For this review, take the finished solid that the model builds, in its own axes (mm). Face numbers are marked on the shaded views. Give positions to 0.01 mm unless a question says otherwise; leave off trailing zeros. Loops run counter-clockwise (first coordinate to the right, second up) from the corner with the lowest first, then second, coordinate; pieces in that order, holes last.
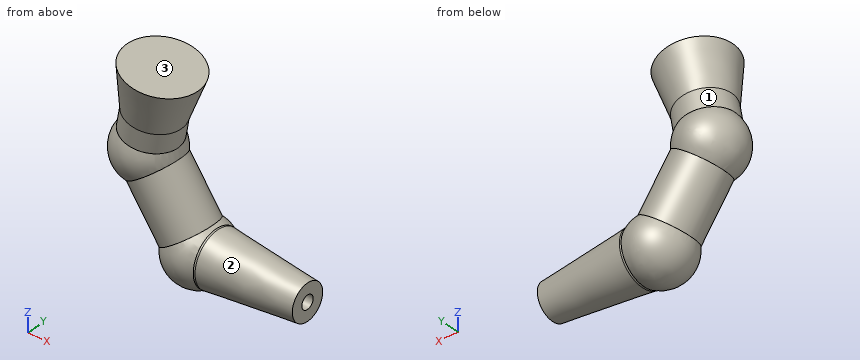
```python
from build123d import *

# Parameters (mm, degrees)
ESQUISSE1_R        = 3
ESQUISSE1_R_2      = 0.75
BOSS_EXTRU_1_DEPTH = 12
CHANFREIN1_SIZE    = 10
CHANFREIN1_SIZE2   = 1
ESQUISSE4_R        = 3
BOSS_EXTRU_2_DEPTH = 10
ESQUISSE8_R        = 3
BOSS_EXTRU_3_DEPTH = 4
ESQUISSE10_R       = 4
BOSS_EXTRU_4_DEPTH = 5
CHANFREIN2_SIZE    = 5
CHANFREIN2_SIZE_2  = 1


with BuildPart() as part:
    # Esquisse1 → Boss.-Extru.1 (new body)
    with BuildSketch(Plane(origin=(0, 0, 0), x_dir=(0, 0, -1), z_dir=(1, 0, 0))):
        Circle(ESQUISSE1_R)
        Circle(ESQUISSE1_R_2, mode=Mode.SUBTRACT)
    extrude(amount=BOSS_EXTRU_1_DEPTH)

    # Chanfrein1
    chanfrein1_edges = [part.edges().sort_by_distance(p)[0] for p in [
        (12, 0, 3),
    ]]
    chanfrein1_side = [part.faces().sort_by_distance(p)[0] for p in [
        (6, 0, 3),
    ]]
    chamfer(chanfrein1_edges, length=CHANFREIN1_SIZE, length2=CHANFREIN1_SIZE2, reference=chanfrein1_side[0])

    # Esquisse2 → Révolution1 (revolve)
    with BuildSketch(Plane.ZY):
        with BuildLine():
            Line((0, 3.5), (0, -3.5))
            ThreePointArc((0, -3.5), (-3.5, 0), (0, 3.5))
        make_face()
    revolve(axis=Axis((0, 3.5, 0), (0, -1, 0)))

    # Esquisse4 → Boss.-Extru.2 (add)
    with BuildSketch(Plane(origin=(0, 0, 0), x_dir=(0, 1, 0), z_dir=(-0.5735764363510443, 0, 0.819152044288993))):
        with Locations(Location((0, 0, 0), (0, 0, 90))):
            Circle(ESQUISSE4_R)
    extrude(amount=BOSS_EXTRU_2_DEPTH)

    # Esquisse7 → Révolution2 (revolve)
    with BuildSketch(Plane(origin=(-5.735764364, 0, 8.191520443), x_dir=(0.8191520442889931, 0, 0.5735764363510444), z_dir=(-0.5735764363510444, 0, 0.8191520442889931))):
        with BuildLine():
            Line((0, 3.5), (0, -3.5))
            ThreePointArc((0, -3.5), (-3.5, 0), (0, 3.5))
        make_face()
    revolve(axis=Axis((-5.735764364, -5.88356871, 8.191520443), (0, 1, 0)))

    # Esquisse8 → Boss.-Extru.3 (add)
    with BuildSketch(Plane(origin=(1.22787804, 0, 6.963642403), x_dir=(0, 1, 0), z_dir=(0.1736481776669342, 0, 0.9848077530122075))):
        with Locations(Location((0, 7.071067812, 0), (0, 0, 90))):
            Circle(ESQUISSE8_R)
    extrude(amount=BOSS_EXTRU_3_DEPTH)

    # Esquisse10 → Boss.-Extru.4 (add)
    with BuildSketch(Plane(origin=(1.92247075, 0, 10.902873415), x_dir=(0.9848077530122075, 0, -0.17364817766693422), z_dir=(0.17364817766693422, 0, 0.9848077530122075))):
        with Locations((-7.071067812, 0)):
            Circle(ESQUISSE10_R)
    extrude(amount=BOSS_EXTRU_4_DEPTH)

    # Chanfrein2
    # the kernel refuses this chamfer: 5, 1 mm, written as the material it takes off along each edge
    with BuildSketch(Plane(origin=(-5.041171653, 0, 12.130751455), x_dir=(0.9848077530122075, 0, -0.17364817766693408), z_dir=(0, -1, 0))) as chanfrein2_piece_1:
        Polygon((4, CHANFREIN2_SIZE), (4 - CHANFREIN2_SIZE_2, 0), (4, 0), align=None)
    revolve(axis=Axis((-5.041171653, 0, 12.130751455), (0.17364817766693422, 0, 0.9848077530122075)), mode=Mode.SUBTRACT)


solid = part.part
```
Item 1: The part is to be moulded in two halves that separate along Z. For the marked faces 1, 2 and 3, say which applies: released by +Z, released by -Z, zero draft, split by the parting line, or undercut.
Answer:
face 1: undercut
face 2: split by the parting line
face 3: released by +Z
Item 2: For L1, parallel to Z at x = 5.75, y = 0 (3 decimals); L2, parallel to Z at x = 10, y = 0; L3, parallel to Y at x = 8.5, z = -0.5, list the stretches that pass through material, from the lowest coordinate up.
Answer:
L1: z = -2.625 to -0.75, 0.75 to 2.625
L2: z = -2.2 to -0.75, 0.75 to 2.2
L3: y = -2.3 to -0.56, 0.56 to 2.3
Item 3: Take a section at A-A on x = 6. Give the boundary of the cut face in (y, z), and give its area (3 significant figures).
Answer:
outline: circle Ø5.2 at (0, 0); hole circle Ø1.5 at (0, 0)
area: 19.5 mm2
Item 4: Take a section at B-B on y = 0. Give the boundary of the cut face in (x, z), and give its area (3 significant figures).
Answer:
outline: (-8.38, 10.49) arc R3.5 ccw to (-7.16, 4.99) - (-3.49, -0.24) arc R3.5 ccw to (1.8, -3) - (2, -3) - (12, -2) - (12, -0.75) - (3.42, -0.75) arc R3.5 ccw to (3.42, 0.75) - (12, 0.75) - (12, 2) - (2, 3) - (1.8, 3) arc R3.5 ccw to (1.42, 3.2) - (-2.24, 8.44) arc R3.5 ccw to (-2.47, 9.45) - (-2.09, 11.61) - (-0.23, 16.36) - (-8.11, 17.75) - (-8, 12.65) - close
area: 173 mm2
Item 5: Clearance check with flat-ended pins moving along their axes: pin 1 Ø1.5 at (y, z) = (-1.5, -1) entering from -X; pin 2 Ø2 at (y, z) = (0, 0) entering from -X; pin 3 Ø5 at (x, z) = (0.5, 10.5) entering from -Y; pin 4 Ø2 at (y, z) = (-2.5, 0) entering from -X. State where each tip first meets the part, or that it passes through.
Answer:
pin 1: stops at x = -3.34
pin 2: stops at x = -4.36
pin 3: passes through
pin 4: stops at x = -3.44
Item 6: Take a section at C-C on z = 9. Give the boundary of the cut face in (x, y).
Answer:
outline: circle Ø6.81 at (-5.74, 0)
